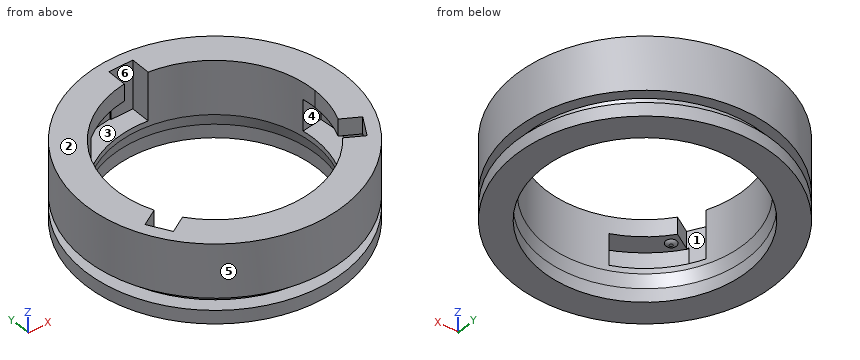
from build123d import *

# Parameters (mm, degrees)
F0_R      = 48
F0_R_2    = 42
F0_R_3    = 38
F1_DEPTH  = 5
F2_R      = 43.0776189128
F2_R_2    = 38
F3_DEPTH  = 4.5
F3_TAPER  = -15
F4_R      = 48.0278860385
F4_R_2    = 44.2833902788
F4_R_3    = 36.7942286341
F5_DEPTH  = 20
F7_DEPTH  = 18
F9_DEPTH  = 11.7
F10_R     = 1.9886860781
F11_DEPTH = 0.73


# Not quite as in the source:
# - a fillet or chamfer that OpenCascade refuses, or shapes differently, is made with other operations: its cross-section is extruded or revolved along the edge and cut away or added


with BuildPart() as f1:
    # F0 (on Top) → F1 (new body)
    with BuildSketch(Plane.XY):
        Circle(F0_R)
        Circle(F0_R_2, mode=Mode.SUBTRACT)
        Circle(F0_R_2)
        Circle(F0_R_3, mode=Mode.SUBTRACT)
    extrude(amount=F1_DEPTH)

    # F2 (on face) → F3 (join)
    with BuildSketch(Plane.XY.offset(5)):
        Circle(F2_R)
        Circle(F2_R_2, mode=Mode.SUBTRACT)
    extrude(amount=F3_DEPTH, taper=F3_TAPER)

    # F4 (on face) → F5 (join)
    with BuildSketch(Plane.XY.offset(9.5)):
        Circle(F4_R)
        Circle(F4_R_2, mode=Mode.SUBTRACT)
        Circle(F4_R_2)
        Circle(F4_R_3, mode=Mode.SUBTRACT)
    extrude(amount=F5_DEPTH)

    # F6 (on face) → F7 (cut)
    with BuildSketch(Plane.XY.offset(29.5)):
        Polygon((4.3897340074, 43.6625890434), (0, 43.6625890434), (-4.3897340074, 43.6625890434), (-4.3897340074, 34.0553857386), (0, 34.0553857386), (4.3897340074, 34.0553857386), align=None)
        Polygon((-35.6180443029, -25.632915688), (-27.2979621816, -20.8293140356), (-29.4928291853, -17.0276928693), (-31.687696189, -13.226071703), (-40.0077783103, -18.0296733554), (-37.8129113066, -21.8312945217), align=None)
        Polygon((40.0077783103, -18.0296733554), (31.687696189, -13.226071703), (29.4928291853, -17.0276928693), (27.2979621816, -20.8293140356), (35.6180443029, -25.632915688), (37.8129113066, -21.8312945217), align=None)
    extrude(amount=-F7_DEPTH, mode=Mode.SUBTRACT)

    # F8 (on face) → F9 (cut)
    with BuildSketch(Plane.XY.offset(11.5)):
        with BuildLine():
            ThreePointArc((-22.6687016251, 28.98180856), (-14.0459580236, 34.0077391776), (-4.3897340074, 36.5314316188))
            Line((-4.3897340074, 36.5314316188), (-4.3897340074, 43.6625890434))
            Line((-4.3897340074, 43.6625890434), (-3.592736461, 43.6625890434))
            Line((-3.592736461, 43.6625890434), (-3.592736461, 44.0917754576))
            ThreePointArc((-3.592736461, 44.0917754576), (-16.0835403712, 41.210582954), (-27.2238685762, 34.869089435))
            Line((-27.2238685762, 34.869089435), (-22.6687016251, 28.98180856))
        make_face()
        with BuildLine():
            ThreePointArc((36.4333332731, 5.1407671981), (36.7038939019, 2.5767097647), (36.7942286341, 0))
            ThreePointArc((36.7942286341, 0), (35.9635026363, -7.7744285261), (33.5088362695, -15.1978009146))
            Line((33.5088362695, -15.1978009146), (39.9809658747, -18.9344866844))
            ThreePointArc((39.9809658747, -18.9344866844), (43.7311819285, -6.6765369327), (43.8094515456, 6.1420170588))
            Line((43.8094515456, 6.1420170588), (36.4333332731, 5.1407671981))
        make_face()
        with BuildLine():
            Line((-16.5855829694, -41.0111064938), (-13.764631648, -34.1225757581))
            ThreePointArc((-13.764631648, -34.1225757581), (-22.7450346913, -28.9219407659), (-29.9160998084, -21.4206030033))
            Line((-29.9160998084, -21.4206030033), (-36.3882294137, -25.1572887731))
            ThreePointArc((-36.3882294137, -25.1572887731), (-27.6476415573, -34.5340460213), (-16.5855829694, -41.0111064938))
        make_face()
    extrude(amount=F9_DEPTH, mode=Mode.SUBTRACT)

    # F10 (on face) → F11 (join)
    with BuildSketch(Plane(origin=(0, 0, 23.2), x_dir=(1, 0, 0), z_dir=(0, 0, -1))):
        with Locations((-30.6445658207, 26.5157744288)):
            Circle(F10_R)
        with Locations((38.2856171667, 13.2810852742)):
            Circle(F10_R)
        with Locations((-7.6410513461, -39.7968597031)):
            Circle(F10_R)
    extrude(amount=F11_DEPTH)

    # F12: fillet of radius 1.6899494937 on 3 edges, made by hand

    # F12_s1 → F12_t2 (revolve, cut)
    with BuildSketch(Plane.XZ.offset(26.5157744288)):
        with BuildLine():
            ThreePointArc((-28.6558797426, 23.2), (-29.2613300231, 22.6635879979), (-30.0467162753, 22.47))
            Line((-30.0467162753, 22.47), (-28.6558797426, 22.47))
            Line((-28.6558797426, 22.47), (-28.6558797426, 23.2))
        make_face()
    revolve(axis=Axis((-30.6445658207, -26.5157744288, 22.47), (0, 0, -1)), mode=Mode.SUBTRACT)

    # F12_s3 → F12_t4 (revolve, cut)
    with BuildSketch(Plane.XZ.offset(13.2810852742)):
        with BuildLine():
            ThreePointArc((40.2743032449, 23.2), (39.6688529644, 22.6635879979), (38.8834667121, 22.47))
            Line((38.8834667121, 22.47), (40.2743032449, 22.47))
            Line((40.2743032449, 22.47), (40.2743032449, 23.2))
        make_face()
    revolve(axis=Axis((38.2856171667, -13.2810852742, 22.47), (0, 0, -1)), mode=Mode.SUBTRACT)

    # F12_s5 → F12_t6 (revolve, cut)
    with BuildSketch(Plane.XZ.offset(-39.7968597031)):
        with BuildLine():
            ThreePointArc((-5.6523652679, 23.2), (-6.2578155484, 22.6635879979), (-7.0432018006, 22.47))
            Line((-7.0432018006, 22.47), (-5.6523652679, 22.47))
            Line((-5.6523652679, 22.47), (-5.6523652679, 23.2))
        make_face()
    revolve(axis=Axis((-7.6410513461, 39.7968597031, 22.47), (0, 0, -1)), mode=Mode.SUBTRACT)


solid = f1.part
The model under review builds one solid part; all positions refer to its coordinate system, in mm. Face numbers are marked on the shaded views. A direction names the side the tool comes from. Round coordinates to 2 decimals unless told otherwise and drop trailing zeros. Order: outer loops, then holes, each group sorted by start corner. A loop starts at its lowest first (then second) coordinate and runs counter-clockwise, first axis right, second up. Notation, with made-up numbers: (-21, -25) -> (26, -25) arc R14 ccw to (26, -11) -> close; hole circle Ø8 at (-35, -12). An arc over 180 degrees is marked (long way). Use CSV: the item, a comma, the result in double quotes. Start each with the question number.
(1) Insertion check: pin 1 (1.5 mm diameter, centred on x = -28.5, z = 16.5, fed in from +Y); pin 2 (10 mm diameter, centred on x = -22, z = 4, fed in from +Y); pin 3 (5 mm diameter, centred on x = 35.5, z = 26, fed in from +Y). Each pin has a flat end and moves straight along its axis. Give the tip position at first contact, or say it passes through.
(2) Mouldability with a two-part tool opening along Z and no side actions: class the marked faces 1, 2 and 3 as pulls with the +Z half, pulls with the -Z half, needs draft (parallel to the pull), parting line crosses it, or undercut.
(3) Wall thickness on probe 1 along Y at (x, z) = (0, 1.4); probe 2 along Y at (x, z) = (0, 20.5); probe 3 along Z at (x, y) = (36.5, -14.5): over which ranges is each line inside the solid? List them lowest first. Write a range as from..to.
(4) Consider section C-C on z = 7.25. Write out the cut boundary in (x, y).
(5) Consider section B-B on x = 0. Write out the cut boundary in (y, z).
(6) Consider section A-A on z = 18. Write out the cut boundary in (x, y), and give its area (3 significant figures).
(7) Tool access review of the marked faces 4, 5 and 6: name each direction out of +Z, -Z, +X, -X, +Y, -Y from which nothing blocks a thin tool from reaching the whole face with its end or side.
Responses:
1,pin 1,"y = 39.2"
1,pin 2,"y = 44.89"
1,pin 3,"y = 34.9"
2,face 1,"needs draft"
2,face 2,"pulls with the +Z half"
2,face 3,"undercut"
3,probe 1,"-48..-38, 38..48"
3,probe 2,"-48.03..-36.79, 43.66..48.03"
3,probe 3,"0..11.5, 23.2..29.5"
4,outline,"circle Ø87.36 at (0, 0); hole circle Ø74.79 at (0, 0)"
5,outline,"(-48.03, 9.5) -> (-44.28, 9.5) -> (-43.08, 5) -> (-48, 5) -> (-48, 0) -> (-38, 0) -> (-38, 5) -> (-36.79, 9.5) -> (-36.79, 29.5) -> (-48.03, 29.5) -> close; (36.79, 9.5) -> (38, 5) -> (38, 0) -> (48, 0) -> (48, 5) -> (43.08, 5) -> (44.28, 9.5) -> (48.03, 9.5) -> (48.03, 29.5) -> (43.66, 29.5) -> (43.66, 11.5) -> (36.79, 11.5) -> close"
6,outline,"circle Ø96.06 at (0, 0); hole (-40.01, -18.03) -> (-36.02, -24.94) -> (-36.39, -25.16) arc R44.24 ccw to (-16.59, -41.01) -> (-13.76, -34.12) arc R36.79 ccw to (29.44, -22.07) -> (35.62, -25.63) -> (39.61, -18.72) -> (39.98, -18.93) arc R44.24 ccw to (43.81, 6.14) -> (36.43, 5.14) arc R36.79 ccw to (4.39, 36.53) -> (4.39, 43.66) -> (-3.59, 43.66) -> (-3.59, 44.09) arc R44.24 ccw to (-27.22, 34.87) -> (-22.67, 28.98) arc R36.79 ccw to (-33.83, -14.46) -> close"
6,area,"2,310 mm²"
7,face 4,"none"
7,face 5,"+Z, -Z"
7,face 6,"+Z"
